Read the model definition and answer for the solid it produces. Units are mm, in the model's axes. A direction names the side the tool comes from. Coordinates: 2 decimals unless noted, no trailing zeros. Loops run counter-clockwise (first coordinate to the right, second up) from the corner with the lowest first, then second, coordinate; pieces in that order, holes last. Notation, with made-up numbers: (6, 58.5) -> (48, 58.5) arc R14 cw to (48, 77.5) -> close; hole circle Ø3 at (-35, 14). An arc over 180 degrees is marked (long way). Answer in a Markdown table with one row per item.
```python
from build123d import *

# Parameters (mm, degrees)
F2_SIZE = 1.2


with BuildPart() as f1:
    # F0 (on Front) → F1 (revolve)
    with BuildSketch(Plane.XZ):
        Polygon((7.5, 52.5), (0, 52.5), (0, -52.5), (7.5, -52.5), (7.5, -37.5), (10.19, -37.5), (10.19, -35), (7.5, -35), (7.5, 35), (10.19, 35), (10.19, 37.5), (7.5, 37.5), align=None)
    revolve(axis=Axis((0, 0, 0.15672), (0, 0, -1)))

    # F2
    f2_edges = [f1.edges().sort_by_distance(p)[0] for p in [
        (-10.19, 0, 37.5),
        (-10.19, 0, -35),
    ]]
    chamfer(f2_edges, length=F2_SIZE)


solid = f1.part
```
1. A tool of negligible diameter and unlimited length cuts with its end or side. For faces 4 (the cylindrical face through (-7.493, -0.33, 45.105)), 5 (the flat face through (1, -8, 35)), 6 (the flat face through (1, -8, -37.5)), 7 (the flat face through (0, 0, 52.5)), 8 (the flat face through (0, 0, -52.5)), from which of +Z, -Z, +X, -X, +Y, -Y can it reach the whole face along a straight path? Write none if from no direction.
A:
| item | result |
|---|---|
| face 4 | +Z |
| face 5 | none |
| face 6 | -Z |
| face 7 | +Z, +X, -X, +Y, -Y |
| face 8 | -Z, +X, -X, +Y, -Y |
2. The mould has two halves that part along Z. Classify faces 1 (the cylindrical face through (-2.209, 9.948, 35.659)), 2 (the flat face through (-5, 6, -35)), 3 (the flat face through (-5, 6, 37.5)): pulls with the +Z half, pulls with the -Z half, needs draft (parallel to the pull), parting line crosses it, or undercut.
A:
| item | result |
|---|---|
| face 1 | needs draft |
| face 2 | undercut |
| face 3 | pulls with the +Z half |
3. A cutting plane is placed at A-A on y = 0. Give the vertices of the cut face in (x, z).
A:
| item | result |
|---|---|
| outline | (-10.19, -37.5) -> (-7.5, -37.5) -> (-7.5, -52.5) -> (7.5, -52.5) -> (7.5, -37.5) -> (10.19, -37.5) -> (10.19, -36.2) -> (8.99, -35) -> (7.5, -35) -> (7.5, 35) -> (10.19, 35) -> (10.19, 36.3) -> (8.99, 37.5) -> (7.5, 37.5) -> (7.5, 52.5) -> (-7.5, 52.5) -> (-7.5, 37.5) -> (-8.99, 37.5) -> (-10.19, 36.3) -> (-10.19, 35) -> (-7.5, 35) -> (-7.5, -35) -> (-8.99, -35) -> (-10.19, -36.2) -> close |
4. Find the intervals of material crossed by probe 1 along Z at (x, y) = (2.25, -7.5); probe 2 along X at (y, z) = (0.25, 4.5); probe 3 along Y at (x, z) = (6.75, 8.5), in increasing order.
A:
| item | result |
|---|---|
| probe 1 | z = -37.5 to -35, 35 to 37.5 |
| probe 2 | x = -7.5 to 7.5 |
| probe 3 | y = -3.27 to 3.27 |
5. A cutting plane is placed at C-C on z = -21.5. Give the vertices of the cut face in (x, y).
A:
| item | result |
|---|---|
| outline | circle Ø15 at (0, 0) |
6. Given pin 1 Ø10 at (x, y) = (8, -7) entering from -Z; pin 2 Ø1 at (x, z) = (0.5, -8.5) entering from -Y; pin 3 Ø8 at (x, z) = (6.5, -0.5) entering from +Y, each flat-ended and moving along its own axis, determine where each tip first touches the part or whether it passes through.
A:
| item | result |
|---|---|
| pin 1 | stops at z = -52.5 |
| pin 2 | stops at y = -7.5 |
| pin 3 | stops at y = 7.07 |
